Work out the finished part from the listing and answer in its coordinate system (mm). Coordinates: 2 decimals unless noted, no trailing zeros. Order: outer loops, then holes, each group sorted by start corner. A loop starts at its lowest first (then second) coordinate and runs counter-clockwise, first axis right, second up. Notation, with made-up numbers: (57.25, 42.25) -> (82.25, 42.25) arc R18 cw to (82.25, 49.25) -> close; hole circle Ø4 at (66.5, -12.5). An arc over 180 degrees is marked (long way). Answer as CSV lines item,"result". Start each with the question number.
Item 1: Section D-D (z = -42) is taken. Write down the section's boundary in (x, y).
Item 2: For a pull along Z with two mould halves and no side action, classify faces 1 (the face through (38.822, 1.288, -63.367)), 2 (the face through (127, 1, -1)), 3 (the face through (14.946, 1.252, -0.099)) as pulls with the +Z half, pulls with the -Z half, needs draft (parallel to the pull), parting line crosses it, or undercut.
Item 3: Straight lines are drawn through the part: L1, parallel to X at y = 2.35, z = 1; L2, parallel to Z at x = 12.5, y = 1.5; L3, parallel to X at y = 1.8, z = -1. For each, find the intervals that lie inside material, in ascending order.
Item 4: Each of these flat-tipped pins is pushed along its axis until it touches: pin 1 Ø4 at (x, z) = (38.1, 0) entering from -Y; pin 2 Ø1 at (x, y) = (70.5, 0.5) entering from -Z; pin 3 Ø1.5 at (y, z) = (2, -40.5) entering from +X. Where does it stop, or does it pass through?
Item 5: Section C-C (y = 2.1) is taken. Write down the section's boundary in (x, z) (3 decimals).
Item 6: Section B-B (z = 0) is taken. Write down the section's boundary in (x, y), then the cut area to 3 significant figures.
Item 7: Section A-A (x = 88.9) is taken. Write down the section's boundary in (y, z), then the cut area to 3 significant figures.
```python
from build123d import *

# Parameters (mm, degrees)
BOSS_EXTRUDE1_DEPTH     = 2.54
F_1_4_CLEARANCE_HOLE1_D = 6.7564
F_8_CLEARANCE_HOLE3_D   = 4.4958
FILLET1_R               = 6.35
SKETCH14_R              = 3.175
CUT_EXTRUDE1_DEPTH      = 2.54


with BuildPart() as part:
    # Sketch1 → Boss-Extrude1 (new body)
    with BuildSketch(Plane(origin=(0, 0, 0), x_dir=(1, 0, 0), z_dir=(0, 1, 0))):
        with BuildLine():
            Line((127, -12.7), (12.7, -12.7))
            ThreePointArc((12.7, -12.7), (4.882201751, -10.008597831), (0.377921481, -3.07512292))
            Line((0.377921481, -3.07512292), (-12.322078519, 47.81402892))
            ThreePointArc((-12.322078519, 47.81402892), (-10.008597831, 58.706950088), (0, 63.58915184))
            Line((0, 63.58915184), (38.85740346, 63.58915184))
            Line((38.85740346, 63.58915184), (127, 12.7))
            Line((127, 12.7), (127, -12.7))
        make_face()
    extrude(amount=BOSS_EXTRUDE1_DEPTH)

    # 1/4 Clearance Hole1 (through all)
    with Locations(Plane(origin=(0, 2.54, 0), x_dir=(1, 0, 0), z_dir=(0, 1, 0))):
        with Locations((0, 43.956848345)):
            Hole(F_1_4_CLEARANCE_HOLE1_D / 2)

    # #8 Clearance Hole3 (through all)
    with Locations(Plane(origin=(0, 2.54, 0), x_dir=(1, 0, 0), z_dir=(0, 1, 0))):
        with Locations((12.7, 0), (38.1, 0), (63.5, 0), (88.9, 0), (114.3, 0)):
            Hole(F_8_CLEARANCE_HOLE3_D / 2)

    # Fillet1
    fillet1_edges = [part.edges().sort_by_distance(p)[0] for p in [
        (127, 1.27, 12.7),
        (38.85740346, 1.27, -63.58915184),
        (127, 1.27, -12.7),
    ]]
    fillet(fillet1_edges, radius=FILLET1_R)

    # Sketch14 → Cut-Extrude1 (cut)
    with BuildSketch(Plane(origin=(0, 2.54, 0), x_dir=(1, 0, 0), z_dir=(0, 1, 0))):
        with Locations(Location((4.83277957, 24.209700029, 0), (0, 0, 270))):
            Circle(SKETCH14_R)
    extrude(amount=-CUT_EXTRUDE1_DEPTH, mode=Mode.SUBTRACT)


solid = part.part
```
Checked values:
1,outline,"(-10.87, 0) -> (-2.75, 0) -> (-2.75, 2.54) -> (-10.87, 2.54) -> close; (2.75, 0) -> (76.25, 0) -> (76.25, 2.54) -> (2.75, 2.54) -> close"
2,face 1,"pulls with the -Z half"
2,face 2,"needs draft"
2,face 3,"undercut"
3,L1,"x = -0.14 to 10.69, 14.71 to 36.09, 40.11 to 61.49, 65.51 to 86.89, 90.91 to 112.29, 116.31 to 127"
3,L2,"z = -63.59 to -2.24, 2.24 to 12.7"
3,L3,"x = -0.64 to 10.69, 14.71 to 36.09, 40.11 to 61.49, 65.51 to 86.89, 90.91 to 112.29, 116.31 to 127"
4,pin 1,"passes through"
4,pin 2,"stops at z = -45.61"
4,pin 3,"stops at x = 80.15"
5,outline,"(-12.322, -47.814) arc R12.7 ccw to (0, -63.589) -> (37.156, -63.589) arc R6.35 ccw to (40.331, -62.738) -> (123.825, -14.533) arc R6.35 ccw to (127, -9.034) -> (127, 6.35) arc R6.35 ccw to (120.65, 12.7) -> (12.7, 12.7) arc R12.7 ccw to (0.378, 3.075) -> close; hole circle Ø6.756 at (0, -43.957); hole circle Ø6.35 at (4.833, -24.21); hole circle Ø4.496 at (12.7, 0); hole circle Ø4.496 at (38.1, 0); hole circle Ø4.496 at (63.5, 0); hole circle Ø4.496 at (88.9, 0); hole circle Ø4.496 at (114.3, 0)"
6,outline,"(-0.39, 0) -> (10.45, 0) -> (10.45, 2.54) -> (-0.39, 2.54) -> close; (14.95, 0) -> (35.85, 0) -> (35.85, 2.54) -> (14.95, 2.54) -> close; (40.35, 0) -> (61.25, 0) -> (61.25, 2.54) -> (40.35, 2.54) -> close; (65.75, 0) -> (86.65, 0) -> (86.65, 2.54) -> (65.75, 2.54) -> close; (91.15, 0) -> (112.05, 0) -> (112.05, 2.54) -> (91.15, 2.54) -> close; (116.55, 0) -> (127, 0) -> (127, 2.54) -> (116.55, 2.54) -> close"
6,area,"266 mm^2"
7,outline,"(0, -34.7) -> (2.54, -34.7) -> (2.54, -2.25) -> (0, -2.25) -> close; (0, 2.25) -> (2.54, 2.25) -> (2.54, 12.7) -> (0, 12.7) -> close"
7,area,"109 mm^2"
